from build123d import *

# Parameters (mm, degrees)
SKIZZE1_R                       = 6.7
SKIZZE1_R_2                     = 3.75
AUFSATZ_LINEAR_AUSTRAGEN1_DEPTH = 9
SKIZZE1_7_R                     = 9.75
SKIZZE1_7_R_2                   = 3.75
AUFSATZ_LINEAR_AUSTRAGEN2_DEPTH = 3
M2_GEWINDEBOHRUNG1_D            = 1.6
SKIZZE5_R                       = 1.05
SCHNITT_LINEAR_AUSTRAGEN1_DEPTH = 13
SKIZZE5_3_R                     = 2
SKIZZE5_3_R_2                   = 1.05
SCHNITT_LINEAR_AUSTRAGEN2_DEPTH = 9


with BuildPart() as part:
    # Skizze1 → Aufsatz-Linear austragen1 (new body)
    with BuildSketch(Plane.XY):
        Circle(SKIZZE1_R)
        Circle(SKIZZE1_R_2, mode=Mode.SUBTRACT)
    extrude(amount=AUFSATZ_LINEAR_AUSTRAGEN1_DEPTH)

    # Skizze1<7> → Aufsatz-Linear austragen2 (add)
    with BuildSketch(Plane.XY):
        Circle(SKIZZE1_7_R)
        Circle(SKIZZE1_7_R_2, mode=Mode.SUBTRACT)
    extrude(amount=-AUFSATZ_LINEAR_AUSTRAGEN2_DEPTH)

    # M2 Gewindebohrung1 (through all)
    with Locations(Plane.XY.offset(9)):
        with Locations((4.425, 0), (0, -4.425), (-4.425, 0), (0, 4.425)):
            Hole(M2_GEWINDEBOHRUNG1_D / 2)

    # Skizze5 → Schnitt-Linear austragen1 (cut, through all)
    with BuildSketch(Plane.XY.offset(9)):
        with Locations((5.409366876, 5.409366876)):
            Circle(SKIZZE5_R)
        with Locations((5.409366876, -5.409366876)):
            Circle(SKIZZE5_R)
        with Locations((-5.409366876, -5.409366876)):
            Circle(SKIZZE5_R)
        with Locations((-5.409366876, 5.409366876)):
            Circle(SKIZZE5_R)
    extrude(amount=-SCHNITT_LINEAR_AUSTRAGEN1_DEPTH, mode=Mode.SUBTRACT)

    # Skizze5<3> → Schnitt-Linear austragen2 (cut)
    with BuildSketch(Plane.XY.offset(9)):
        with Locations((-5.409366876, 5.409366876)):
            Circle(SKIZZE5_3_R)
        with Locations((-5.409366876, 5.409366876)):
            Circle(SKIZZE5_3_R_2, mode=Mode.SUBTRACT)
        with Locations((5.409366876, 5.409366876)):
            Circle(SKIZZE5_3_R)
        with Locations((5.409366876, 5.409366876)):
            Circle(SKIZZE5_3_R_2, mode=Mode.SUBTRACT)
        with Locations((5.409366876, -5.409366876)):
            Circle(SKIZZE5_3_R)
        with Locations((5.409366876, -5.409366876)):
            Circle(SKIZZE5_3_R_2, mode=Mode.SUBTRACT)
        with Locations((-5.409366876, -5.409366876)):
            Circle(SKIZZE5_3_R)
        with Locations((-5.409366876, -5.409366876)):
            Circle(SKIZZE5_3_R_2, mode=Mode.SUBTRACT)
    extrude(amount=-SCHNITT_LINEAR_AUSTRAGEN2_DEPTH, mode=Mode.SUBTRACT)


solid = part.part
Source: CAD feature listing. Evaluate the final solid. Frame: model axes, mm. A direction names the side the tool comes from. Coordinates: 2 decimals unless noted, no trailing zeros. Order: outer loops, then holes, each group sorted by start corner. A loop starts at its lowest first (then second) coordinate and runs counter-clockwise, first axis right, second up. Notation, with made-up numbers: M -35.75,35 L 22.25,35 A8 cw 22.25,43 Z; hole C 20.25,77.25 d11. An arc over 180 degrees is marked long. Write each question's results on one line, items separated by ' | '. Start each with the question number.
1. Material intervals for L1, parallel to Z at x = 2.5, y = 7.5; L2, parallel to X at y = 4.25, z = 1.25; L3, parallel to Y at x = -3, z = 0.75, sorted ascending.
2. Section D-D, the plane z = -0.75. Return the cut outline in (x, y) (3 decimals), then the cut area to 3 significant figures.
3. Reachability of faces 1 (the face through (-6.7, 0.1, 4.4)), 2 (the face through (3.98, 4.01, 4.56)), 3 (the face through (2.7, 2.6, 3.1)), 4 (the face through (4, -2, -3)), 5 (the face through (-0.1, -6.7, 4.4)) from +Z, -Z, +X, -X, +Y, -Y: full face, straight path, thin tool, end or side. Return the list, or none.
4. Draft query along Y for faces 6 (the face through (4.01, -3.98, 4.56)), 7 (the face through (6.7, -0.1, 4.4)), 8 (the face through (3, -3, 9)). Return one class per face: +Y half, -Y half, draft (parallel to the pull), parting line (faces both ways), or undercut.
5. Section C-C, the plane z = 7. Return the cut outline in (x, y) (3 decimals), then the cut area to 3 significant figures.
6. Pin query (flat end, axial travel): pin 1 (1.5 mm diameter, centred on x = -0.5, y = 3, fed in from +Z); pin 2 (6 mm diameter, centred on x = -8, z = 6.5, fed in from +Y); pin 3 (6 mm diameter, centred on y = 7, z = -1, fed in from -X); pin 4 (6 mm diameter, centred on x = 2, z = 6, fed in from -Y). Return the tip coordinate at first contact, or that it passes through.
7. Section A-A, the plane x = 0. Return the cut outline in (y, z) (3 decimals), then the cut area to 3 significant figures.
Solution:
1) L1: -3 to 0 | L2: -3.78 to -0.78, 0.78 to 3.78 | L3: -5.99 to -2.25, 2.25 to 5.99
2) outline: C 0,0 d19.5; hole C -5.409,-5.409 d2.1; hole C -5.409,5.409 d2.1; hole M -3.729,-0.395 A3.75 ccw -0.395,-3.729 A0.8 ccw long 0.395,-3.729 A3.75 ccw 3.729,-0.395 A0.8 ccw long 3.729,0.395 A3.75 ccw 0.395,3.729 A0.8 ccw long -0.395,3.729 A3.75 ccw -3.729,0.395 A0.8 ccw long Z; hole C 5.409,-5.409 d2.1; hole C 5.409,5.409 d2.1 | area: 233 mm²
3) face 1: +Z, -X | face 2: +Z | face 3: +Z, -Z | face 4: -Z, +X, -X, +Y, -Y | face 5: +Z, -Y
4) face 6: undercut | face 7: parting line | face 8: draft
5) outline: M -5.75,-3.439 A2 cw -3.439,-5.75 A6.7 ccw 3.439,-5.75 A2 cw 5.75,-3.439 A6.7 ccw 5.75,3.439 A2 cw 3.439,5.75 A6.7 ccw -3.439,5.75 A2 cw -5.75,3.439 A6.7 ccw Z; hole M -3.729,-0.395 A3.75 ccw -0.395,-3.729 A0.8 ccw long 0.395,-3.729 A3.75 ccw 3.729,-0.395 A0.8 ccw long 3.729,0.395 A3.75 ccw 0.395,3.729 A0.8 ccw long -0.395,3.729 A3.75 ccw -3.729,0.395 A0.8 ccw long Z | area: 79.5 mm²
6) pin 1: z = 9 | pin 2: y = 3.45 | pin 3: x = -8.89 | pin 4: y = -6.7
7) outline: M -9.75,-3 L -5.225,-3 L -5.225,9 L -6.7,9 L -6.7,0 L -9.75,0 Z; M 5.225,-3 L 9.75,-3 L 9.75,0 L 6.7,0 L 6.7,9 L 5.225,9 Z | area: 53.7 mm²
